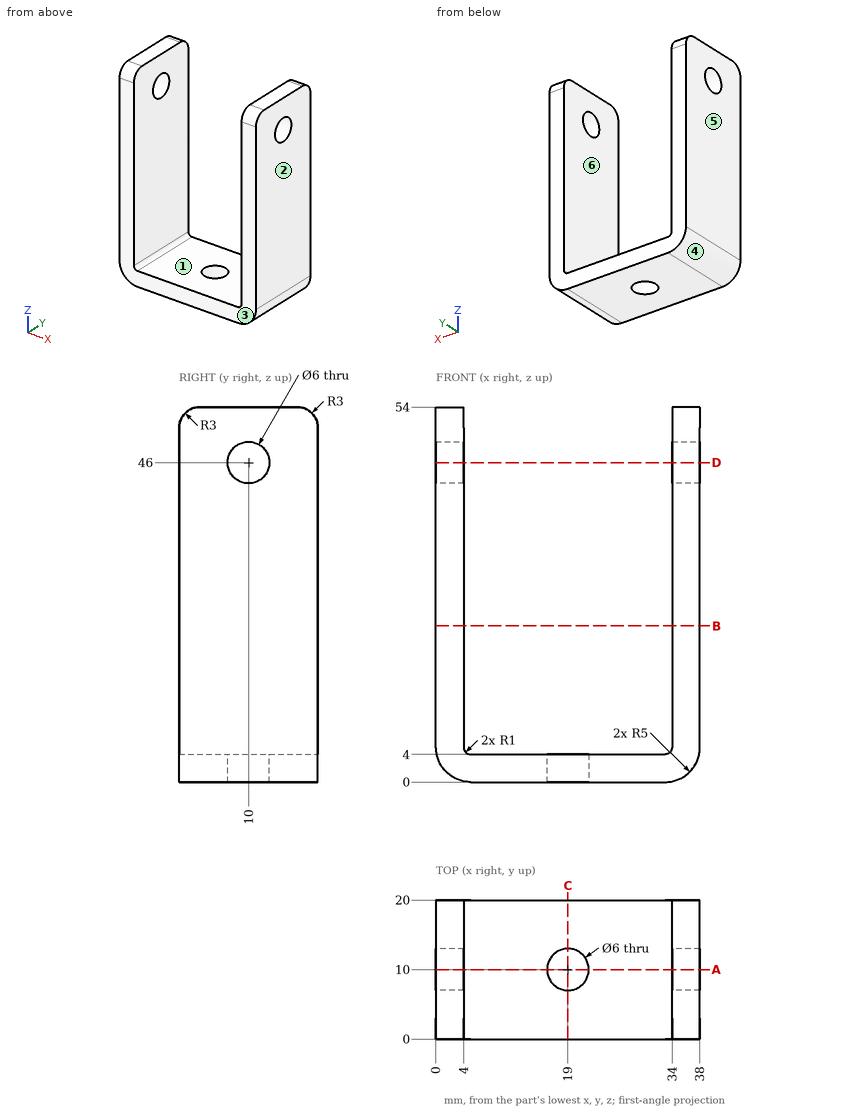
Part print with two shaded views. Sizes in mm from the minimum x, y, z corner. A direction names the side the tool comes from. Coordinates: 2 decimals unless noted, no trailing zeros. Write each loop counter-clockwise with the first axis right and the second up, starting at its lowest first coordinate (ties: lowest second). Pieces come first, ordered by that corner, then holes.
(1) Drill centre lines: line 1 (X direction, y = 17, z = 42); line 2 (Y direction, x = 2.95, z = 46); line 3 (Z direction, x = 26.5, y = 14.75). Where is each one in solid material? Low to high.
(2) Cut at D-D on z = 46. List the corners of the cut face in (x, y).
(3) Pin check, flat tips, straight feed: pin 1 Ø6 at (x, y) = (17.5, 13) entering from +Z; pin 2 Ø6 at (x, z) = (7.5, 23) entering from -Y. Stop position of each tip, or through.
(4) 3-axis set-ups, long thin cutter, end or side, ignore diameter. For the marked faces 5 and 6: which of +Z, -Z, +X, -X, +Y, -Y reach the whole face in a straight line?
(5) Cut at C-C on x = 19. List the corners of the cut face in (y, z), and give its area (3 significant figures).
(6) Cut at B-B on z = 22.5. List the corners of the cut face in (x, y).
(7) Mould opens along X. For the marked faces 1, 2, 3 and 4 say: pulls with the +X half, pulls with the -X half, needs draft (parallel to the pull), parting line crosses it, or undercut.
(8) Cut at A-A on y = 10. List the corners of the cut face in (x, z).
Working result:
1. line 1: x = 0 to 4, 34 to 38
1. line 2: y = 0 to 7, 13 to 20
1. line 3: z = 0 to 4
2. outline: (0, 0) - (4, 0) - (4, 7) - (0, 7) - close; (0, 13) - (4, 13) - (4, 20) - (0, 20) - close; (34, 0) - (38, 0) - (38, 7) - (34, 7) - close; (34, 13) - (38, 13) - (38, 20) - (34, 20) - close
3. pin 1: stops at z = 4
3. pin 2: passes through
4. face 5: +Z, -Z, -X, +Y, -Y
4. face 6: +Z, +Y, -Y
5. outline: (0, 0) - (7, 0) - (7, 4) - (0, 4) - close; (13, 0) - (20, 0) - (20, 4) - (13, 4) - close
5. area: 56.0 mm2
6. outline: (0, 0) - (4, 0) - (4, 20) - (0, 20) - close; (34, 0) - (38, 0) - (38, 20) - (34, 20) - close
7. face 1: undercut
7. face 2: pulls with the +X half
7. face 3: needs draft
7. face 4: pulls with the -X half
8. outline: (0, 5) arc R5 ccw to (5, 0) - (16, 0) - (16, 4) - (5, 4) arc R1 cw to (4, 5) - (4, 43) - (0, 43) - close; (0, 49) - (4, 49) - (4, 54) - (0, 54) - close; (22, 0) - (33, 0) arc R5 ccw to (38, 5) - (38, 43) - (34, 43) - (34, 5) arc R1 cw to (33, 4) - (22, 4) - close; (34, 49) - (38, 49) - (38, 54) - (34, 54) - close
